Input: part model. Units: mm. Frame: model coordinates. Face numbers are marked on the shaded views. Coordinates: 2 decimals unless noted, no trailing zeros. Write each loop counter-clockwise with the first axis right and the second up, starting at its lowest first coordinate (ties: lowest second). Pieces come first, ordered by that corner, then holes. Notation, with made-up numbers: (-28, 89.5) - (-5, 89.5) arc R31 ccw to (-5, 120.5) - close; hole circle Ø6 at (88, -27). An arc over 180 degrees is marked (long way). Use CSV: the item, a comma, the result in double quotes.
```python
from build123d import *

# Parameters (mm, degrees)
SKETCH1_R           = 2.05
BOSS_EXTRUDE1_DEPTH = 2
BOSS_EXTRUDE2_DEPTH = 8
FILLET2_R           = 1


with BuildPart() as part:
    # Sketch1 → Boss-Extrude1 (new body)
    with BuildSketch(Plane(origin=(0, 0, 0), x_dir=(1, 0, 0), z_dir=(0, 1, 0))):
        with BuildLine():
            Line((1.8, 0), (38.2, 0))
            ThreePointArc((38.2, 0), (39.472792206, 0.527207794), (40, 1.8))
            Line((40, 1.8), (40, 18.2))
            ThreePointArc((40, 18.2), (39.472792206, 19.472792206), (38.2, 20))
            Line((38.2, 20), (1.8, 20))
            ThreePointArc((1.8, 20), (0.527207794, 19.472792206), (0, 18.2))
            Line((0, 18.2), (0, 1.8))
            ThreePointArc((0, 1.8), (0.527207794, 0.527207794), (1.8, 0))
        make_face()
        with Locations(Location((10, 10, 0), (0, 0, 270))):
            Circle(SKETCH1_R, mode=Mode.SUBTRACT)
        with Locations(Location((30, 10, 0), (0, 0, 270))):
            Circle(SKETCH1_R, mode=Mode.SUBTRACT)
    extrude(amount=BOSS_EXTRUDE1_DEPTH)

    # Sketch1_2 → Boss-Extrude2 (add)
    with BuildSketch(Plane(origin=(0, 0, 0), x_dir=(1, 0, 0), z_dir=(0, 1, 0))):
        with BuildLine():
            ThreePointArc((7.95, 10), (10, 7.95), (12.05, 10))
            Line((12.05, 10), (7.95, 10))
        make_face()
        with BuildLine():
            Line((7.95, 10), (12.05, 10))
            ThreePointArc((12.05, 10), (10, 12.05), (7.95, 10))
        make_face()
        with BuildLine():
            ThreePointArc((27.95, 10), (30, 7.95), (32.05, 10))
            Line((32.05, 10), (27.95, 10))
        make_face()
        with BuildLine():
            Line((27.95, 10), (32.05, 10))
            ThreePointArc((32.05, 10), (30, 12.05), (27.95, 10))
        make_face()
    extrude(amount=BOSS_EXTRUDE2_DEPTH)

    # Fillet1: read off the stored shape, not the designer's step
    # Fillet1 outline → Fillet1 (revolve, cut)
    with BuildSketch(Plane(origin=(10, 0, -10), x_dir=(1, 0, 0), z_dir=(0, 0, 1))):
        with BuildLine():
            ThreePointArc((0.05, 8), (1.464213562, 7.414213562), (2.05, 6))
            Line((2.05, 6), (2.05, 8))
            Line((2.05, 8), (0.05, 8))
        make_face()
    revolve(axis=Axis((10, 0, -10), (0, 1, 0)), mode=Mode.SUBTRACT)

    # Fillet1 2 outline → Fillet1 2 (revolve, cut)
    with BuildSketch(Plane(origin=(30, 0, -10), x_dir=(1, 0, 0), z_dir=(0, 0, 1))):
        with BuildLine():
            ThreePointArc((0.05, 8), (1.464213562, 7.414213562), (2.05, 6))
            Line((2.05, 6), (2.05, 8))
            Line((2.05, 8), (0.05, 8))
        make_face()
    revolve(axis=Axis((30, 0, -10), (0, 1, 0)), mode=Mode.SUBTRACT)

    # Fillet2
    fillet2_edges = [part.edges().sort_by_distance(p)[0] for p in [
        (20, 0, 0),
        (0.527207794, 0, -0.527207794),
        (0, 0, -10),
        (0.527207794, 0, -19.472792206),
        (20, 0, -20),
        (39.472792206, 0, -19.472792206),
        (40, 0, -10),
        (39.472792206, 0, -0.527207794),
    ]]
    fillet(fillet2_edges, radius=FILLET2_R)


solid = part.part
```
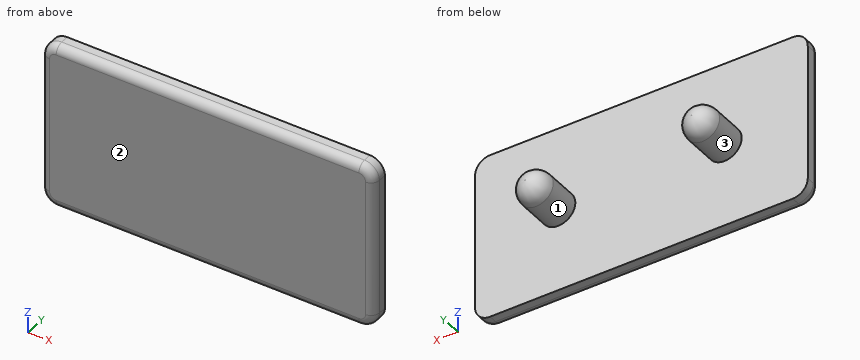
(1) Ray query, probe 1 along Y at (x, z) = (29, -17.5); probe 2 along X at (y, z) = (6.75, -10.75); probe 3 along X at (y, z) = (3.5, -10). Return the intervals inside material, ascending. Write a range as from..to.
Check values:
probe 1,"0..2"
probe 2,"8.25..11.75, 28.25..31.75"
probe 3,"7.95..12.05, 27.95..32.05"
(2) Draft query along X for the marked faces 1, 2 and 3. Return one class per face: pulls with the +X half, pulls with the -X half, needs draft (parallel to the pull), parting line crosses it, or undercut.
Check values:
face 1,"undercut"
face 2,"needs draft"
face 3,"undercut"
(3) Cut plane B-B on x = 7. Return loops of the section in (y, z), and give its area (3 significant figures).
Check values:
outline,"(0, -19) arc R1 ccw to (1, -20) - (2, -20) - (2, 0) - (1, 0) arc R1 ccw to (0, -1) - close"
area,"39.6 mm^2"
(4) Cut plane A-A on y = 3.5. Return loops of the section in (x, z).
Check values:
outline,"circle Ø4.1 at (10, -10); circle Ø4.1 at (30, -10)"
(5) Cut plane C-C on z = -16.5. Return loops of the section in (x, y), and give its area (3 significant figures).
Check values:
outline,"(0, 1) arc R1 ccw to (1, 0) - (39, 0) arc R1 ccw to (40, 1) - (40, 2) - (0, 2) - close"
area,"79.6 mm^2"
(6) Pin query (flat end, axial travel): pin 1 Ø6 at (x, z) = (27, -6.5) entering from +Y. Return the tip coordinate at first contact, or that it passes through.
Check values:
pin 1,"y = 7.25"
